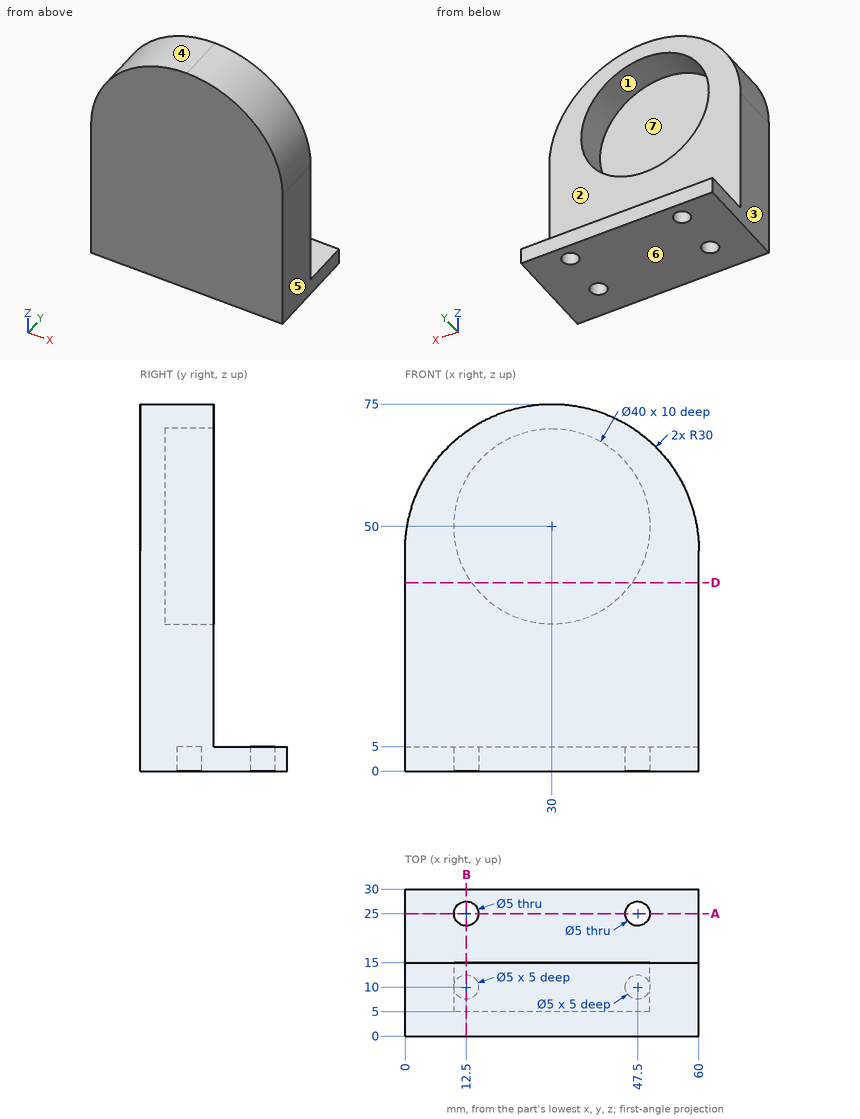
Input: dimensioned drawing with shaded views. Units: mm. Origin: part minimum x, y, z. A direction names the side the tool comes from. Coordinates: 2 decimals unless noted, no trailing zeros. Write each loop counter-clockwise with the first axis right and the second up, starting at its lowest first coordinate (ties: lowest second). Pieces come first, ordered by that corner, then holes. Notation, with made-up numbers: M -27.75,-28 L -14.75,-28 A29 ccw -14.75,5 Z; hole C 39,59 d3. An arc over 180 degrees is marked long. Use a Markdown table: item, result.
1) Reachability of the marked faces 1, 2 and 3 from +Z, -Z, +X, -X, +Y, -Y: full face, straight path, thin tool, end or side. Return the list, or none.
Conclusion:
| item | result |
|---|---|
| face 1 | +Y |
| face 2 | +Z, +X, -X, +Y |
| face 3 | +Z, -Z, -X, +Y, -Y |
2) Section B-B, the plane x = 12.5. Output: boundary loops of the cut face in (y, z), then the cut area to 3 significant figures.
Conclusion:
| item | result |
|---|---|
| outline | M 0,0 L 7.5,0 L 7.5,5 L 12.5,5 L 12.5,0 L 22.5,0 L 22.5,5 L 15,5 L 15,40.32 L 5,40.32 L 5,59.68 L 15,59.68 L 15,69.37 L 0,69.37 Z; M 27.5,0 L 30,0 L 30,5 L 27.5,5 Z |
| area | 872 mm^2 |
3) Mould query, pull axis Z, two halves, no side actions, for the marked faces 4, 5, 6 and 7. Classes: pulls with the +Z half, pulls with the -Z half, needs draft (parallel to the pull), parting line crosses it, or undercut.
Conclusion:
| item | result |
|---|---|
| face 4 | pulls with the +Z half |
| face 5 | needs draft |
| face 6 | pulls with the -Z half |
| face 7 | undercut |
4) Ray query, L1, parallel to Y at x = 47.5, z = 3.1; L2, parallel to Y at x = 12, z = 2; L3, parallel to Y at x = 57.5, z = 44. Return the intervals inside material, ascending.
Conclusion:
| item | result |
|---|---|
| L1 | y = 0 to 7.5, 12.5 to 22.5, 27.5 to 30 |
| L2 | y = 0 to 7.55, 12.45 to 22.55, 27.45 to 30 |
| L3 | y = 0 to 15 |
5) Section D-D, the plane z = 38.5. Output: boundary loops of the cut face in (x, y), then the cut area to 3 significant figures.
Conclusion:
| item | result |
|---|---|
| outline | M 0,0 L 60,0 L 60,15 L 46.36,15 L 46.36,5 L 13.64,5 L 13.64,15 L 0,15 Z |
| area | 573 mm^2 |
6) First-contact query: pin 1 Ø10 at (y, z) = (19.5, 52) entering from -X; pin 2 Ø20 at (x, z) = (31.5, 43) entering from +Y; pin 3 Ø1.5 at (x, y) = (47.5, 9.5) entering from -Z. Flat tips, straight axial feed; report the tip coordinate or a pass-through.
Conclusion:
| item | result |
|---|---|
| pin 1 | stops at x = 0.39 |
| pin 2 | stops at y = 5 |
| pin 3 | stops at z = 5 |
7) Section A-A, the plane y = 25. Output: boundary loops of the cut face in (x, z).
Conclusion:
| item | result |
|---|---|
| outline | M 0,0 L 10,0 L 10,5 L 0,5 Z; M 15,0 L 45,0 L 45,5 L 15,5 Z; M 50,0 L 60,0 L 60,5 L 50,5 Z |
